```python
from build123d import *

# Parameters (mm, degrees)
SKETCH1_W           = 70
SKETCH1_H           = 200
BOSS_EXTRUDE1_DEPTH = 80
FILLET1_R           = 10
SKETCH2_R           = 24.442521079
BOSS_EXTRUDE2_DEPTH = 15
FILLET3_R           = 10
SKETCH3_R           = 12
BOSS_EXTRUDE3_DEPTH = 50
SKETCH4_R           = 30
BOSS_EXTRUDE4_DEPTH = 20
FILLET4_R           = 10
SKETCH5_R           = 10
CUT_EXTRUDE1_DEPTH  = 80


with BuildPart() as part:
    # Sketch1 → Boss-Extrude1 (new body)
    with BuildSketch(Plane.XY):
        with Locations((20.223475334, 1.448561813)):
            Rectangle(SKETCH1_W, SKETCH1_H)
    extrude(amount=BOSS_EXTRUDE1_DEPTH)

    # Fillet1
    fillet1_edges = [part.edges().sort_by_distance(p)[0] for p in [
        (55.223475334, 1.448561813, 80),
        (20.223475334, 101.448561813, 80),
        (-14.776524666, 1.448561813, 80),
        (20.223475334, 101.448561813, 0),
        (55.223475334, 1.448561813, 0),
        (20.223475334, -98.551438187, 0),
        (-14.776524666, 1.448561813, 0),
        (-14.776524666, 101.448561813, 40),
        (55.223475334, 101.448561813, 40),
        (55.223475334, -98.551438187, 40),
        (-14.776524666, -98.551438187, 40),
        (20.223475334, -98.551438187, 80),
    ]]
    fillet(fillet1_edges, radius=FILLET1_R)

    # Sketch2 → Boss-Extrude2 (add)
    with BuildSketch(Plane(origin=(0, -98.551438187, 0), x_dir=(-1, 0, 0), z_dir=(0, -1, 0))):
        with Locations((-20.223475334, -40)):
            Circle(SKETCH2_R)
    extrude(amount=BOSS_EXTRUDE2_DEPTH)

    # Fillet3
    fillet3_edges = [part.edges().sort_by_distance(p)[0] for p in [
        (44.665996414, -113.551438187, 40),
    ]]
    fillet(fillet3_edges, radius=FILLET3_R)

    # Sketch3 → Boss-Extrude3 (add)
    with BuildSketch(Plane.XZ.offset(113.551438187)):
        with Locations((20.19472106, 39.984491152)):
            Circle(SKETCH3_R)
    extrude(amount=BOSS_EXTRUDE3_DEPTH)

    # Sketch4 → Boss-Extrude4 (add)
    with BuildSketch(Plane(origin=(0, -163.551438187, 0), x_dir=(-1, 0, 0), z_dir=(0, -1, 0))):
        with Locations((-20.19472106, -39.984491152)):
            Circle(SKETCH4_R)
    extrude(amount=BOSS_EXTRUDE4_DEPTH)

    # Fillet4
    fillet4_edges = [part.edges().sort_by_distance(p)[0] for p in [
        (50.19472106, -163.551438187, 39.984491152),
    ]]
    fillet(fillet4_edges, radius=FILLET4_R)

    # Sketch5 → Cut-Extrude1 (cut)
    with BuildSketch(Plane.XY.offset(80)):
        with Locations((20.223475334, 56.448561813)):
            Circle(SKETCH5_R)
        with Locations((20.223475334, 26.448561813)):
            Circle(SKETCH5_R)
        with Locations((20.223475334, -3.551438187)):
            Circle(SKETCH5_R)
    extrude(amount=-CUT_EXTRUDE1_DEPTH, mode=Mode.SUBTRACT)


solid = part.part
```
Read the model definition and answer for the solid it produces. Units are mm, in the model's axes. A direction names the side the tool comes from. Coordinates: 2 decimals unless noted, no trailing zeros. Loops run counter-clockwise (first coordinate to the right, second up) from the corner with the lowest first, then second, coordinate; pieces in that order, holes last. Notation, with made-up numbers: (4, -0.5) -> (59, -0.5) arc R20 ccw to (59, 23.5) -> close; hole circle Ø10 at (39, -29). An arc over 180 degrees is marked (long way). Return JSON: item names as keys, results as strings.
Item 1: Find the intervals of material crossed by probe 1 along Y at (x, z) = (20, 52.5); probe 2 along X at (y, z) = (27.5, 63.5); probe 3 along Y at (x, z) = (15.5, 70), in increasing order.
Answers:
{"probe 1": "y = -183.55 to -163.55, -113.55 to -13.55, 6.45 to 16.45, 36.45 to 46.45, 66.45 to 101.45", "probe 2": "x = -14.78 to 10.28, 30.17 to 55.22", "probe 3": "y = -98.55 to -12.37, 5.26 to 17.63, 35.26 to 47.63, 65.26 to 101.45"}
Item 2: For faces 1 (the cylindrical face through (-11.925, 2.709, 3.007)), 2 (the cylindrical face through (26.7, -178.48, 69.27)), 3 (the cylindrical face through (17.59, -138.2, 28.27)), 4 (the cylindrical face through (-11.925, -95.544, 40.42)), determine the directions among +Z, -Z, +X, -X, +Y, -Y from which every point of the face is accessible in a straight line to the end or side of a thin tool.
Answers:
{"face 1": "-Z, -X, +Y, -Y", "face 2": "-Y", "face 3": "none", "face 4": "+Z, -Z, -X"}
Item 3: A flat-ended cylindrical pin translates along its axis: P1, Ø1.5, axis at x = 32, y = -115, coming from the +Z side. Find the tip coordinate at first contact, or state that the pin passes through.
Answers:
{"P1": "stops at z = 44.65"}
Item 4: Find section C-C (y = -94). Determine the outline of the cut face in (x, z).
Answers:
{"outline": "(-13.16, 10) arc R8.39 ccw to (-4.78, 1.61) -> (45.22, 1.61) arc R8.39 ccw to (53.61, 10) -> (53.61, 70) arc R8.39 ccw to (45.22, 78.39) -> (-4.78, 78.39) arc R8.39 ccw to (-13.16, 70) -> close"}
Item 5: Find section A-A (y = -41.5). Determine the outline of the cut face in (x, z), plus the area to 3 significant figures.
Answers:
{"outline": "(-14.78, 10) arc R10 ccw to (-4.78, 0) -> (45.22, 0) arc R10 ccw to (55.22, 10) -> (55.22, 70) arc R10 ccw to (45.22, 80) -> (-4.78, 80) arc R10 ccw to (-14.78, 70) -> close", "area": "5,510 mm2"}
Item 6: Find section D-D (y = -154). Determine the outline of the cut face in (x, z).
Answers:
{"outline": "circle Ø24 at (20.19, 39.98)"}
Item 7: Find section B-B (z = 35). Count the separate pieces of the cut face and the enclosed holes in it, plus the area to 3 significant figures.
Answers:
{"separate pieces": "1", "enclosed holes": "3", "area": "15,900 mm2"}
Item 8: For a pull along X with two mould halves and no side action, classify faces 5 (the cylindrical face through (-3.09, -101.02, 32.66)), 6 (the cylindrical face through (20.57, -95.7, 3.01)), 7 (the cylindrical face through (18.056, 16.686, 40.56)) as +X half, -X half, draft (parallel to the pull), parting line (faces both ways), or undercut.
Answers:
{"face 5": "parting line", "face 6": "draft", "face 7": "undercut"}
